Source: CAD feature listing. Evaluate the final solid. Frame: model axes, mm. Give positions to 0.01 mm unless a question says otherwise; leave off trailing zeros. Order: outer loops, then holes, each group sorted by start corner. A loop starts at its lowest first (then second) coordinate and runs counter-clockwise, first axis right, second up. Notation, with made-up numbers: M 59.25,-21.5 L 70.25,-21.5 A22 cw 70.25,-6.5 Z; hole C -35,51.5 d3. An arc over 180 degrees is marked long. Return JSON: item names as keys, results as strings.
Autodesk Inventor part; units mm, degrees
ref_plane "YZ Plane" through (0, 0, 0) normal (1, 0, 0) x (0, 1, 0)
ref_plane "XZ Plane" through (0, 0, 0) normal (0, 1, 0) x (-1, 0, 0)
ref_plane "XY Plane" through (0, 0, 0) normal (0, 0, 1) x (1, 0, 0)
sketch "Sketch1" plane through (0, 0, 0) normal (0, 0, 1) x (1, 0, 0)
  line L0 (5, -7.5) -> (-5, -7.5) construction
  line L1 (-5, -7.5) -> (-5, 7.5) construction
  line L2 (-5, 7.5) -> (5, 7.5) construction
  line L3 (5, 7.5) -> (5, -7.5) construction
  line L4 (5, -7.5) -> (-5, 7.5) construction
  line L5 (-5, -7.5) -> (5, 7.5) construction
  line L6 (0, 0) -> (21.2132, -21.2132) construction
  line L7 (0, 0) -> (-17.3205, -10) construction
  line L8 (-20.5912, -7.6973) -> (-8.2707, 9.8027)
  arc A0 (-5, 11.5) -> (-8.2707, 9.8027) centre (-5, 7.5) ccw
  line L9 (-5, 11.5) -> (5, 11.5)
  arc A1 (8.4831, 9.4668) -> (5, 11.5) centre (5, 7.5) ccw
  line L10 (8.4831, 9.4668) -> (24.6963, -19.2464)
  arc A2 (20.0956, -25.0539) -> (24.6963, -19.2464) centre (21.2132, -21.2132) ccw
  line L11 (20.0956, -25.0539) -> (-18.4381, -13.8407)
  arc A3 (-20.5912, -7.6973) -> (-18.4381, -13.8407) centre (-17.3205, -10) ccw
  dimension "d0" = 10
  dimension "d1" = 15
  dimension "d2" = 30
  dimension "d4" = 45
  dimension "d5" = 30
  dimension "d6" = 20
  dimension "d7" = 4
extrude "Extrusion1" add sketch "Sketch1" against normal blind 3
hole "Hole1" at (-5, 7.5, 0) at (5, 7.5, 0) at (5, -7.5, 0) at (-5, -7.5, 0) direction (0, 0, -1) diameter 3 depth 8 tip angle 118
hole "Hole2" at (-17.3205, -10, 0) at (21.2132, -21.2132, 0) direction (0, 0, -1) diameter 3 depth 8 tip angle 118
hole "Hole3" at (0, 0, 0) direction (0, 0, -1) diameter 3 depth 8 tip angle 118
properties part number "LegBase_front"
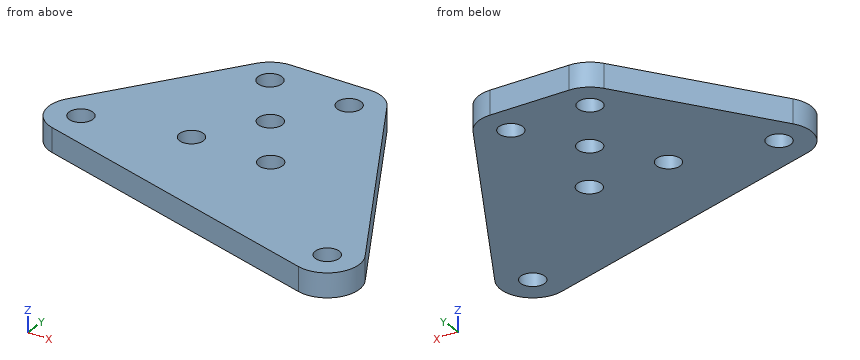
1. Ray query, probe 1 along X at (y, z) = (7, -0.3); probe 2 along X at (y, z) = (-7.5, -0.65); probe 3 along Y at (x, z) = (5, -1.1). Return the intervals inside material, ascending.
Evaluation:
{"probe 1": "x = -10.24 to -6.41, -3.59 to 3.59, 6.41 to 9.88", "probe 2": "x = -20.45 to -6.5, -3.5 to 3.5, 6.5 to 18.06", "probe 3": "y = -20.66 to -9, -6 to 6, 9 to 11.5"}
2. First-contact query: pin 1 (1.8 mm diameter, centred on x = 0, y = 0, fed in from -Z); pin 2 (1 mm diameter, centred on y = -2, z = -0.5, fed in from -X); pin 3 (1.5 mm diameter, centred on x = -6, z = -2.5, fed in from -Y); pin 4 (1 mm diameter, centred on x = -15, z = -2, fed in from -Y). Flat tips, straight axial feed; report the tip coordinate or a pass-through.
Evaluation:
{"pin 1": "passes through", "pin 2": "stops at x = -16.93", "pin 3": "stops at y = -17.68", "pin 4": "stops at y = -14.99"}
3. Section query A-A (y = 7.5). Return loops of the section in (x, z), then the cut area to 3 significant figures.
Evaluation:
{"outline": "M -9.89,-3 L -6.5,-3 L -6.5,0 L -9.89,0 Z; M -3.5,-3 L 3.5,-3 L 3.5,0 L -3.5,0 Z; M 6.5,-3 L 9.59,-3 L 9.59,0 L 6.5,0 Z", "area": "40.5 mm^2"}
4. Section query B-B (x = 22). Return loops of the section in (y, z).
Evaluation:
{"outline": "M -25.14,-3 L -22.49,-3 L -22.49,0 L -25.14,0 Z; M -19.94,-3 L -14.47,-3 L -14.47,0 L -19.94,0 Z"}
5. Section query C-C (y = -10). Return loops of the section in (x, z), then the cut area to 3 significant figures.
Evaluation:
{"outline": "M -21.32,-3 L -18.82,-3 L -18.82,0 L -21.32,0 Z; M -15.82,-3 L 19.48,-3 L 19.48,0 L -15.82,0 Z", "area": "113 mm^2"}
6. Section query D-D (z = -2). Return loops of the section in (x, y), then the cut area to 3 significant figures.
Evaluation:
{"outline": "M -20.59,-7.7 A4 ccw -18.44,-13.84 L 20.1,-25.05 A4 ccw 24.7,-19.25 L 8.48,9.47 A4 ccw 5,11.5 L -5,11.5 A4 ccw -8.27,9.8 Z; hole C -17.32,-10 d3; hole C -5,-7.5 d3; hole C -5,7.5 d3; hole C 0,0 d3; hole C 5,-7.5 d3; hole C 5,7.5 d3; hole C 21.21,-21.21 d3", "area": "969 mm^2"}
